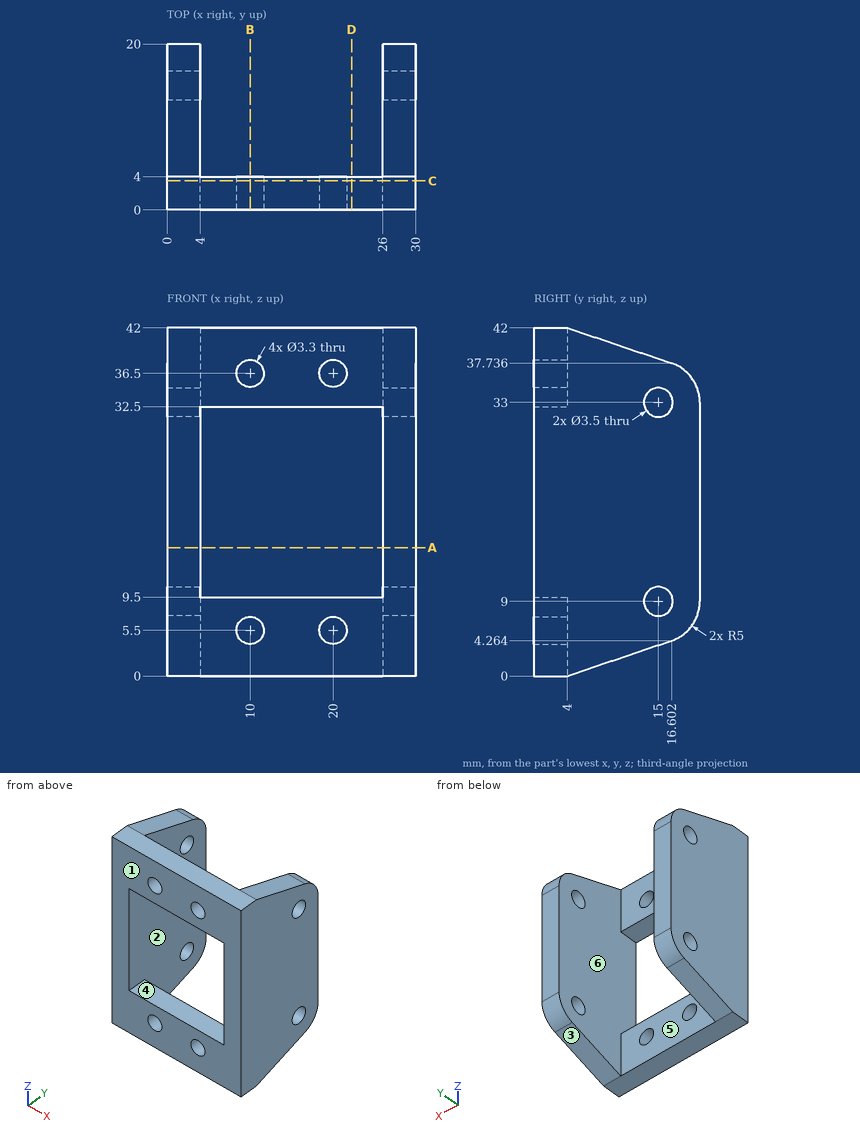
Source: three-view drawing plus pictorial views. Frame: mm from the lowest corner of the part. A direction names the side the tool comes from. Coordinates: 2 decimals unless noted, no trailing zeros. Order: outer loops, then holes, each group sorted by start corner. A loop starts at its lowest first (then second) coordinate and runs counter-clockwise, first axis right, second up.
Item 1: Set-up query: the marked faces 4, 5 and 6. Return all of +Z, -Z, +X, -X, +Y, -Y with unobstructed straight access to the full face (end or side cutting, diameter ignored); none if empty.
Output values:
face 4: +Y, -Y
face 5: +Z, -Z, +Y
face 6: +Y
Item 2: Pull-direction query (Z, two-part tool) for the marked faces 1, 2 and 3; classes: pulls with the +Z half, pulls with the -Z half, needs draft (parallel to the pull), parting line crosses it, or undercut.
Output values:
face 1: needs draft
face 2: undercut
face 3: pulls with the -Z half
Item 3: Cut plane D-D (x = 22.25). Return loops of the section in (y, z), plus the area to 3 significant figures.
Output values:
outline: (0, 0) - (4, 0) - (4, 9.5) - (0, 9.5) - close; (0, 32.5) - (4, 32.5) - (4, 42) - (0, 42) - close
area: 76.0 mm2
Item 4: Material intervals for line 1 (Z direction, x = 20, y = 3.1); line 2 (X direction, y = 1.3, z = 5.5); line 3 (X direction, y = 17.25, z = 31.5), sorted ascending.
Output values:
line 1: z = 0 to 3.85, 7.15 to 9.5, 32.5 to 34.85, 38.15 to 42
line 2: x = 0 to 8.35, 11.65 to 18.35, 21.65 to 30
line 3: x = 0 to 4, 26 to 30
Item 5: Cut plane C-C (y = 3.5). Return loops of the section in (x, z), plus the area to 3 significant figures.
Output values:
outline: (0, 0) - (30, 0) - (30, 42) - (0, 42) - close; hole (4, 9.5) - (26, 9.5) - (26, 32.5) - (4, 32.5) - close; hole circle Ø3.3 at (10, 5.5); hole circle Ø3.3 at (10, 36.5); hole circle Ø3.3 at (20, 5.5); hole circle Ø3.3 at (20, 36.5)
area: 720 mm2
Item 6: Cut plane A-A (z = 15.5). Return loops of the section in (x, y), plus the area to 3 significant figures.
Output values:
outline: (0, 0) - (4, 0) - (4, 20) - (0, 20) - close; (26, 0) - (30, 0) - (30, 20) - (26, 20) - close
area: 160 mm2
Item 7: Cut plane B-B (x = 10). Return loops of the section in (y, z).
Output values:
outline: (0, 0) - (4, 0) - (4, 3.85) - (0, 3.85) - close; (0, 7.15) - (4, 7.15) - (4, 9.5) - (0, 9.5) - close; (0, 32.5) - (4, 32.5) - (4, 34.85) - (0, 34.85) - close; (0, 38.15) - (4, 38.15) - (4, 42) - (0, 42) - close
Item 8: First-contact query: P1, Ø10.5, axis at x = 14, z = 35.5, coming from the +Y side. Flat tip, straight axial feed; report the tip coordinate or a pass-through.
Output values:
P1: stops at y = 4
